```python
from build123d import *

# Parameters (mm, degrees)
F1_DEPTH = 26.4
F2_R     = 2.65
F3_DEPTH = 32.25
F4_DEPTH = 40
F5_W     = 20
F5_H     = 13.16
F6_DEPTH = 4.45
F7_W     = 3.045
F7_H     = 3.15
F8_DEPTH = 20


# Not quite as in the source:
# - a feature names something its author has since deleted; it is built from what else it names


with BuildPart() as f1:
    # F0 (on Front) → F1 (new body)
    with BuildSketch(Plane.XZ):
        Polygon((-12.7175080026, 22.9085270187), (-21.5175080026, 22.9085270187), (-21.5175080026, -15.5114729813), (16.3324919974, -15.5114729813), (16.3324919974, -3.2914729813), (11.3324919974, -3.2914729813), (6.6349683525, -6.7779857958), (0.1349683525, -6.7779857958), (-7.2175080026, 0), (-12.7175080026, 0), align=None)
    extrude(amount=F1_DEPTH)

    # F2 (on face) → F3 (cut)
    with BuildSketch(Plane.XY.offset(22.9085270187)):
        with Locations((-17.1175080026, -4.97)):
            Circle(F2_R)
        with Locations((-17.1175080026, -21.43)):
            Circle(F2_R)
    extrude(amount=-F3_DEPTH, mode=Mode.SUBTRACT)

    # F2 (on face) → F4 (cut)
    with BuildSketch(Plane.XY.offset(22.9085270187)):
        with Locations((-17.1175080026, -13.2)):
            Circle(F2_R)
    extrude(amount=-F4_DEPTH, mode=Mode.SUBTRACT)

    # F5 (on face) → F6 (cut)
    with BuildSketch(Plane(origin=(0, 0, -15.5114729813), x_dir=(1, 0, 0), z_dir=(0, 0, -1))):
        with Locations((6.3324919974, 13.2)):
            Rectangle(F5_W, F5_H)
    extrude(amount=-F6_DEPTH, mode=Mode.SUBTRACT)

    # F7 (on face) → F8 (cut)
    with BuildSketch(Plane.YZ.offset(16.3324919974)):
        with Locations((-5.0975, -12.6364729813)):
            Rectangle(F7_W, F7_H)
        with Locations((-21.3025, -12.6364729813)):
            Rectangle(F7_W, F7_H)
    extrude(amount=-F8_DEPTH, mode=Mode.SUBTRACT)


solid = f1.part
```
Geometry check sheet. Reference: the model listing, model coordinates, mm. A direction names the side the tool comes from. Coordinates: 2 decimals unless noted, no trailing zeros. Loops run counter-clockwise (first coordinate to the right, second up) from the corner with the lowest first, then second, coordinate; pieces in that order, holes last.
Item 1: Sectioned sample at B-B, the plane y = -8.75. Record the boundary of the cut face in (x, z).
Item 2: Access from +Z, -Z, +X, -X, +Y, -Y to the whole of each face (thin tool, end or side, straight path). Record for faces 4 (the face through (6, -19.78, -15)), 5 (the face through (-19.22, -23.04, 7.01)), 6 (the face through (6, -21, -14.211)), 7 (the face through (14, -13, -3.291)), 8 (the face through (3, -13, -6.778)).
Item 3: Thickness scan on line 1 (Y direction, x = -3.5, z = -11.5) (3 decimals); line 2 (Z direction, x = -9.5, y = -15.25); line 3 (X direction, y = -21.25, z = -13). Record the ranges inside material, lowest first.
Item 4: Release check for a two-part mould opening along Y. For faces 1 (the face through (-10, -13, 0)), 2 (the face through (-7, 0, -5)), 3 (the face through (6, -3.575, -13)) record: released by +Y, released by -Y, zero draft, split by the parting line, or undercut.
Item 5: Sectioned sample at D-D, the plane y = -13.2. Record the boundary of the cut face in (x, z), then the cut area to 3 significant figures.
Item 6: Sectioned sample at C-C, the plane x = 2.5. Record the boundary of the cut face in (y, z) (3 decimals).
Item 7: Go/stop test with flat-tipped pins: pin 1 Ø4 at (x, y) = (0, -14.5) entering from -Z; pin 2 Ø8 at (x, z) = (-1.5, 0.5) entering from +Y; pin 3 Ø8.5 at (x, y) = (-17.12, -13.2) entering from +Z; pin 4 Ø7 at (x, y) = (2.5, -18.5) entering from +Z. Record where each tip stops, or that it passes through.
Item 8: Sectioned sample at A-A, the plane z = 10. Record the boundary of the cut face in (x, y), then the cut area to 3 significant figures.
Check result:
1. outline: (-21.52, -15.51) - (-3.67, -15.51) - (-3.67, -11.06) - (16.33, -11.06) - (16.33, -3.29) - (11.33, -3.29) - (6.63, -6.78) - (0.13, -6.78) - (-7.22, 0) - (-12.72, 0) - (-12.72, 22.91) - (-21.52, 22.91) - close
2. face 4: -Z, +X
2. face 5: +Z
2. face 6: +X
2. face 7: +Z, +X, +Y, -Y
2. face 8: +Z, +Y, -Y
3. line 1: y = -26.4 to -22.825, -3.575 to 0
3. line 2: z = -15.51 to 0
3. line 3: x = -21.52 to -3.67
4. face 1: zero draft
4. face 2: released by +Y
4. face 3: undercut
5. outline: (-21.52, -15.51) - (-19.77, -15.51) - (-19.77, 22.91) - (-21.52, 22.91) - close; (-14.47, -15.51) - (-3.67, -15.51) - (-3.67, -11.06) - (16.33, -11.06) - (16.33, -3.29) - (11.33, -3.29) - (6.63, -6.78) - (0.13, -6.78) - (-7.22, 0) - (-12.72, 0) - (-12.72, 22.91) - (-14.47, 22.91) - close
5. area: 387 mm2
6. outline: (-26.4, -15.511) - (-19.78, -15.511) - (-19.78, -14.211) - (-22.825, -14.211) - (-22.825, -11.061) - (-3.575, -11.061) - (-3.575, -14.211) - (-6.62, -14.211) - (-6.62, -15.511) - (0, -15.511) - (0, -6.778) - (-26.4, -6.778) - close
7. pin 1: stops at z = -11.06
7. pin 2: passes through
7. pin 3: stops at z = 22.91
7. pin 4: stops at z = -5.73
8. outline: (-21.52, -26.4) - (-12.72, -26.4) - (-12.72, 0) - (-21.52, 0) - close; hole circle Ø5.3 at (-17.12, -21.43); hole circle Ø5.3 at (-17.12, -13.2); hole circle Ø5.3 at (-17.12, -4.97)
8. area: 166 mm2
